from build123d import *

# Parameters (mm, degrees)
SZKIC1_R                    = 4
DODANIE_WYCI_GNI_CIE1_DEPTH = 40
SZKIC2_R                    = 5
DODANIE_WYCI_GNI_CIE2_DEPTH = 5
ZAOKR_GLENIE1_R             = 5
DODANIE_WYCI_GNI_CIE3_START = 5
SZKIC3_R                    = 5
DODANIE_WYCI_GNI_CIE3_DEPTH = 5
ZAOKR_GLENIE2_R             = 5


with BuildPart() as part:
    # Szkic1 → Dodanie-wyciągnięcie1 (new body)
    with BuildSketch(Plane(origin=(0, 0, 0), x_dir=(1, 0, 0), z_dir=(0, 1, 0))):
        with Locations(Location((0, 0, 0), (0, 0, 270))):
            Circle(SZKIC1_R)
    extrude(amount=DODANIE_WYCI_GNI_CIE1_DEPTH)

    # Szkic2 → Dodanie-wyciągnięcie2 (add)
    with BuildSketch(Plane(origin=(0, 40, 0), x_dir=(1, 0, 0), z_dir=(0, 1, 0))):
        with Locations(Location((0, 0, 0), (0, 0, 270))):
            Circle(SZKIC2_R)
    extrude(amount=DODANIE_WYCI_GNI_CIE2_DEPTH)

    # Zaokrąglenie1
    zaokr_glenie1_edges = [part.edges().sort_by_distance(p)[0] for p in [
        (0, 45, -5),
    ]]
    fillet(zaokr_glenie1_edges, radius=ZAOKR_GLENIE1_R - 0.0001)  # a hair under: the kernel refuses the full size

    # Szkic3 → Dodanie-wyciągnięcie3 (add)
    with BuildSketch(Plane.XZ.offset(DODANIE_WYCI_GNI_CIE3_START)):
        with Locations(Location((0, 0, 0), (0, 0, 270))):
            Circle(SZKIC3_R)
    extrude(amount=-DODANIE_WYCI_GNI_CIE3_DEPTH)

    # Zaokrąglenie2
    zaokr_glenie2_edges = [part.edges().sort_by_distance(p)[0] for p in [
        (0, -5, 5),
    ]]
    fillet(zaokr_glenie2_edges, radius=ZAOKR_GLENIE2_R - 0.0001)  # a hair under: the kernel refuses the full size


solid = part.part
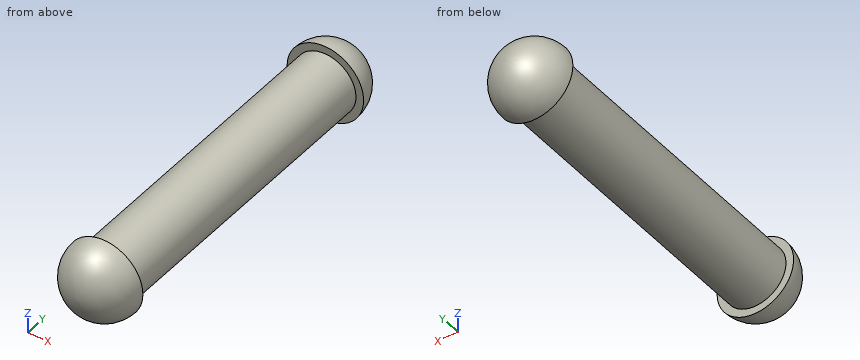
Here's how the part is built. I have some questions about the finished solid (model axes, mm). Round coordinates to 2 decimals unless told otherwise and drop trailing zeros. Order: outer loops, then holes, each group sorted by start corner. A loop starts at its lowest first (then second) coordinate and runs counter-clockwise, first axis right, second up. Notation, with made-up numbers: (66, 14) -> (121, 14) arc R22 cw to (121, 51) -> close; hole circle Ø10 at (8, 29). An arc over 180 degrees is marked (long way). Return JSON: item names as keys, results as strings.
Q1. I need wall thicknesses on line 1 along Y through (x, z) = (-3.25, 3); line 2 along X through (y, z) = (36.5, 0). Which ranges of each line are inside material? Lowest first, please. Write a range as from..to.
Filled sheet:
{"line 1": "y = -2.33..0, 40..42.33", "line 2": "x = -4..4"}
Q2. If we section it at A-A on y = 21: List the corners of the cut face in (x, z) for me, plus the area to 3 significant figures.
Filled sheet:
{"outline": "circle Ø8 at (0, 0)", "area": "50.3 mm^2"}
Q3. For pin 1 Ø4 at (x, z) = (-3, 0.5) entering from +Y; pin 2 Ø4 at (x, z) = (0, 2.5) entering from +Y; pin 3 Ø3 at (x, z) = (0.5, 3.5) entering from +Y, each with a flat end and sliding along its axis, tell me the tip position at first contact or that it passes through.
Filled sheet:
{"pin 1": "stops at y = 44.89", "pin 2": "stops at y = 44.97", "pin 3": "stops at y = 44.57"}
